Check sheet for the modelled part. Datum: model origin and axes. Units: mm. A direction names the side the tool comes from. Give positions to 0.01 mm unless a question says otherwise; leave off trailing zeros. Order: outer loops, then holes, each group sorted by start corner. A loop starts at its lowest first (then second) coordinate and runs counter-clockwise, first axis right, second up. Notation, with made-up numbers: (21, 70.25) -> (58, 70.25) arc R16 cw to (58, 91.25) -> close; hole circle Ø10 at (47.5, 58). An arc over 180 degrees is marked (long way). One line per question, with ' | ' between items.
```python
from build123d import *

# Parameters (mm, degrees)
SKETCH1_W           = 117.475
SKETCH1_H           = 69.85
BOSS_EXTRUDE1_DEPTH = 25.4
SKETCH2_W           = 19.716181521
SKETCH2_H           = 69.85
SKETCH2_W_2         = 17.25680248
CUT_EXTRUDE2_DEPTH  = 15.24
SKETCH3_W           = 44.45
SKETCH3_H           = 31.75
CUT_EXTRUDE4_DEPTH  = 2.54


with BuildPart() as part:
    # Sketch1 → Boss-Extrude1 (new body)
    with BuildSketch(Plane(origin=(0, 0, 0), x_dir=(1, 0, 0), z_dir=(0, 1, 0))):
        with Locations((58.7375, 34.925)):
            Rectangle(SKETCH1_W, SKETCH1_H)
    extrude(amount=BOSS_EXTRUDE1_DEPTH)

    # Sketch2 → Cut-Extrude2 (cut)
    with BuildSketch(Plane(origin=(0, 25.4, 0), x_dir=(1, 0, 0), z_dir=(0, 1, 0))):
        with Locations((9.858090761, 34.925)):
            Rectangle(SKETCH2_W, SKETCH2_H)
        with Locations((108.84659876, 34.925)):
            Rectangle(SKETCH2_W_2, SKETCH2_H)
    extrude(amount=-CUT_EXTRUDE2_DEPTH, mode=Mode.SUBTRACT)

    # Sketch3 → Cut-Extrude4 (cut)
    with BuildSketch(Plane(origin=(0, 25.4, 0), x_dir=(1, 0, 0), z_dir=(0, 1, 0))):
        with Locations((59.96718952, 34.925)):
            Rectangle(SKETCH3_W, SKETCH3_H)
    extrude(amount=-CUT_EXTRUDE4_DEPTH, mode=Mode.SUBTRACT)


solid = part.part
```
Q1. Section check C-C (y = 21). Enter the section's corners in (x, z), and give its area (3 significant figures).
Result sheet:
outline: (19.72, -69.85) -> (100.22, -69.85) -> (100.22, 0) -> (19.72, 0) -> close | area: 5,620 mm2
Q2. Access from +Z, -Z, +X, -X, +Y, -Y to the whole of each face (thin tool, end or side, straight path). Record for faces 4 (the face through (0, 5, -34)), 5 (the face through (19.716, 18, -34)), 6 (the face through (60, 22.86, -35)), 7 (the face through (100.218, 18, -34)).
Result sheet:
face 4: +Z, -Z, -X, +Y, -Y | face 5: +Z, -Z, -X, +Y | face 6: +Y | face 7: +Z, -Z, +X, +Y
Q3. Mould release check, pull along X, two halves, no side actions. Record for faces 1 (the face through (58, 13, 0)), 2 (the face through (37.742, 24, -35)), 3 (the face through (117.475, 5, -34)): pulls with the +X half, pulls with the -X half, needs draft (parallel to the pull), parting line crosses it, or undercut.
Result sheet:
face 1: needs draft | face 2: undercut | face 3: pulls with the +X half
Q4. Section check B-B (x = 40). Enter the section's corners in (y, z).
Result sheet:
outline: (0, -69.85) -> (25.4, -69.85) -> (25.4, -50.8) -> (22.86, -50.8) -> (22.86, -19.05) -> (25.4, -19.05) -> (25.4, 0) -> (0, 0) -> close
Q5. Section check A-A (z = -33.5). Enter the section's corners in (x, y) (3 decimals), and give its area (3 significant figures).
Result sheet:
outline: (0, 0) -> (117.475, 0) -> (117.475, 10.16) -> (100.218, 10.16) -> (100.218, 25.4) -> (82.192, 25.4) -> (82.192, 22.86) -> (37.742, 22.86) -> (37.742, 25.4) -> (19.716, 25.4) -> (19.716, 10.16) -> (0, 10.16) -> close | area: 2,310 mm2
Q6. Section check D-D (z = -15.5). Enter the section's corners in (x, y) (3 decimals), and give its area (3 significant figures).
Result sheet:
outline: (0, 0) -> (117.475, 0) -> (117.475, 10.16) -> (100.218, 10.16) -> (100.218, 25.4) -> (19.716, 25.4) -> (19.716, 10.16) -> (0, 10.16) -> close | area: 2,420 mm2
Q7. Thickness scan on line 1 (Y direction, x = 101.5, z = -21.5); line 2 (X direction, y = 12.25, z = -46.5); line 3 (Y direction, x = 50.5, z = -26). Record the ranges inside material, lowest first.
Result sheet:
line 1: y = 0 to 10.16 | line 2: x = 19.72 to 100.22 | line 3: y = 0 to 22.86
Q8. Depth check by flat-ended pin: pin 1 Ø4.5 at (y, z) = (19.5, -21) entering from -X; pin 2 Ø8 at (y, z) = (15.5, -56) entering from +X; pin 3 Ø6 at (x, z) = (103.5, -46) entering from +Y. Enter the tip coordinate at first touch or a pass-through.
Result sheet:
pin 1: stops at x = 19.72 | pin 2: stops at x = 100.22 | pin 3: stops at y = 10.16
